Verification items for the finished model (mm, model axes). A direction names the side the tool comes from. Round coordinates to 2 decimals unless told otherwise and drop trailing zeros. Loops run counter-clockwise (first coordinate to the right, second up) from the corner with the lowest first, then second, coordinate; pieces in that order, holes last. Notation, with made-up numbers: (-18, 22.25) -> (-4, 22.25) arc R22 ccw to (-4, 40.25) -> close; hole circle Ø6 at (-11.5, 53). An arc over 180 degrees is marked (long way). Write item = value, one per line.
```python
from build123d import *

# Parameters (mm, degrees)
FILLET004_R = 3
FILLET005_R = 1


with BuildPart() as part:
    # Sketch010 → Revolution (revolve)
    with BuildSketch(Plane.XZ):
        with BuildLine():
            Line((0, 79.2), (4.2, 79.2))
            Line((4.2, 79.2), (4.2, 29.2))
            Line((4.2, 29.2), (11.1, 29.2))
            Line((11.1, 29.2), (11.1, 14.2))
            Line((11.1, 14.2), (12.8, 14.2))
            Line((12.8, 14.2), (12.8, 7))
            Line((12.8, 7), (82.8, 7))
            Line((82.8, 7), (82.8, 10))
            Line((82.8, 10), (16.2, 10))
            Line((16.2, 10), (16.2, 83))
            ThreePointArc((16.2, 83), (11.45513, 94.45513), (0, 99.2))
            Line((0, 79.2), (0, 99.2))
        make_face()
    revolve(axis=Axis((0, 0, 0), (0, 0, 1)))

    # Fillet004
    fillet004_edges = [part.edges().sort_by_distance(p)[0] for p in [
        (-16.2, 0, 10),
    ]]
    fillet(fillet004_edges, radius=FILLET004_R)

    # Fillet005
    fillet005_edges = [part.edges().sort_by_distance(p)[0] for p in [
        (-82.8, 0, 10),
        (-82.8, 0, 7),
    ]]
    fillet(fillet005_edges, radius=FILLET005_R)


solid = part.part
```
(1) Sectioned sample at A-A, the plane z = 68.5. Record the cut outline in (x, y), and give its area (3 significant figures).
Filled sheet:
outline = circle Ø32.4 at (0, 0); hole circle Ø8.4 at (0, 0)
area = 769 mm2
(2) Material ranges on probe 1 along Y at (x, z) = (0, 9); probe 2 along Y at (x, z) = (0, 45); probe 3 along X at (y, z) = (-0.5, 45), recorded low to high. Write a range as from..to.
Filled sheet:
probe_1 = -82.8..-12.8, 12.8..82.8
probe_2 = -16.2..-4.2, 4.2..16.2
probe_3 = -16.19..-4.17, 4.17..16.19
(3) Go/stop test with flat-tipped pins: pin 1 Ø1.5 at (x, y) = (-63.5, 5.5) entering from +Z; pin 2 Ø1 at (x, z) = (5, 47.5) entering from -Y; pin 3 Ø6.5 at (x, y) = (0, 0) entering from -Z. Record where each tip stops, or that it passes through.
Filled sheet:
pin_1 = 10
pin_2 = -15.56
pin_3 = 79.2
(4) Set-up check for faces 1 (the face through (4.006, 1.262, 53.85)), 2 (the face through (-3.512, -15.815, 48.49)): record each of +Z, -Z, +X, -X, +Y, -Y from which the full face is reachable in a straight line by a thin tool's end or side.
Filled sheet:
face_1 = -Z
face_2 = +Z
(5) Draft check along Y on faces 3 (the face through (-65.71, -50.38, 8.51)), 4 (the face through (-17, 1, 7)), 5 (the face through (-10.158, -7.789, 10.55)), 6 (the face through (10, 6, 14.2)). Enter one of: released by +Y, released by -Y, zero draft, split by the parting line, or undercut.
Filled sheet:
face_3 = split by the parting line
face_4 = zero draft
face_5 = undercut
face_6 = undercut
